```python
from build123d import *

# Parameters (mm, degrees)
SKETCH1_W           = 113
SKETCH1_H           = 98
BOSS_EXTRUDE1_DEPTH = 100
CUT_EXTRUDE1_DEPTH  = 130
CUT_EXTRUDE3_DEPTH  = 95
SKETCH4_W           = 113
SKETCH4_H           = 88.876192891
CUT_EXTRUDE4_DEPTH  = 95
BOSS_EXTRUDE4_DEPTH = 5
SKETCH7_W           = 36.687301185
SKETCH7_H           = 28.468155535
BOSS_EXTRUDE6_DEPTH = 25
SKETCH8_R           = 15
CUT_EXTRUDE5_DEPTH  = 25
FILLET1_R           = 20


with BuildPart() as part:
    # Sketch1 → Boss-Extrude1 (new body)
    with BuildSketch(Plane(origin=(0, 0, 0), x_dir=(1, 0, 0), z_dir=(0, 1, 0))):
        with Locations((9.126923077, -28.796153846)):
            Rectangle(SKETCH1_W, SKETCH1_H)
    extrude(amount=-BOSS_EXTRUDE1_DEPTH)

    # Sketch2 → Cut-Extrude1 (cut)
    with BuildSketch(Plane(origin=(65.626923077, 0, 0), x_dir=(0, 0, -1), z_dir=(1, 0, 0))):
        Polygon((20.203846154, 0), (-77.796153846, -50), (-77.796153846, 0), align=None)
    extrude(amount=-CUT_EXTRUDE1_DEPTH, mode=Mode.SUBTRACT)

    # Sketch3 → Cut-Extrude3 (cut)
    with BuildSketch(Plane(origin=(0, 0, -20.203846154), x_dir=(-1, 0, 0), z_dir=(0, 0, -1))):
        Polygon((-34.397311681, 0), (47.373076923, -88.732184402), (47.373076923, 0), align=None)
    extrude(amount=-CUT_EXTRUDE3_DEPTH, mode=Mode.SUBTRACT)

    # Sketch4 → Cut-Extrude4 (cut)
    with BuildSketch(Plane(origin=(0, 0, 0), x_dir=(1, 0, 0), z_dir=(0, 1, 0))):
        with Locations((9.126923077, -30.184844361)):
            Rectangle(SKETCH4_W, SKETCH4_H)
    extrude(amount=-CUT_EXTRUDE4_DEPTH, mode=Mode.SUBTRACT)

    # Sketch6 → Boss-Extrude4 (add)
    with BuildSketch(Plane(origin=(65.626923077, 0, 0), x_dir=(0, 0, -1), z_dir=(1, 0, 0))):
        Polygon((14.253252085, -95), (14.253252085, -3.036017382), (-74.622940806, -58.738358676), (-74.622940806, -95), align=None)
    extrude(amount=-BOSS_EXTRUDE4_DEPTH)

    # Sketch7 → Boss-Extrude6 (add)
    with BuildSketch(Plane(origin=(0, -95, 0), x_dir=(1, 0, 0), z_dir=(0, 1, 0))):
        with Locations((42.283272485, 0.019174318)):
            Rectangle(SKETCH7_W, SKETCH7_H)
    extrude(amount=BOSS_EXTRUDE6_DEPTH)

    # Sketch8 → Cut-Extrude5 (cut)
    with BuildSketch(Plane.XY.offset(77.796153846)):
        with Locations((-26.771199052, -75)):
            Circle(SKETCH8_R)
    extrude(amount=-CUT_EXTRUDE5_DEPTH, mode=Mode.SUBTRACT)

    # Fillet1
    # the kernel refuses this fillet: 20 mm, written as the material it takes off along each edge
    with BuildSketch(Plane(origin=(-47.373076923, -25.745870671, 30.258060361), x_dir=(0, -0.8907618697082329, -0.454470341687874), z_dir=(0, -0.45447034168787404, 0.890761869708233))) as fillet1_piece_1:
        with BuildLine():
            CenterArc((FILLET1_R, FILLET1_R), FILLET1_R, 180, 90)
            Line((0, FILLET1_R), (0, 0))
            Line((0, 0), (FILLET1_R, 0))
        make_face()
    extrude(amount=103.367903479, mode=Mode.SUBTRACT)


solid = part.part
```
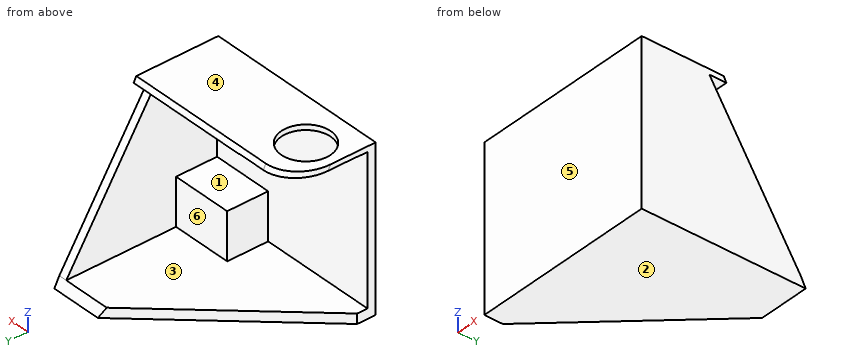
Geometry: final body of the model. Coordinates: model frame, mm. Face numbers are marked on the shaded views. A direction names the side the tool comes from. Round coordinates to 2 decimals unless told otherwise and drop trailing zeros. Order: outer loops, then holes, each group sorted by start corner. A loop starts at its lowest first (then second) coordinate and runs counter-clockwise, first axis right, second up. Notation, with made-up numbers: (37.25, 67.25) -> (70.25, 67.25) arc R18 ccw to (70.25, 84.25) -> close; hole circle Ø8 at (-12, 16). An arc over 180 degrees is marked (long way). Use one line per item in the form item = value. Start each with the question number.
1. Cut plane B-B (x = -31). Return the cut outline in (y, z).
2. Cut plane A-A (y = -75). Return the cut outline in (x, z), then the cut area to 3 significant figures.
3. Reachability of the marked faces 1 and 2 from +Z, -Z, +X, -X, +Y, -Y: full face, straight path, thin tool, end or side. Return the list, or none.
4. Pin query (flat end, axial travel): pin 1 Ø2 at (x, z) = (-18, 17.5) entering from +Y; pin 2 Ø12 at (x, y) = (31, -33.5) entering from +Z; pin 3 Ø12 at (y, z) = (-21, 15) entering from -X. Return the tip coordinate at first contact, or that it passes through.
5. Draft query along Z for the marked faces 3, 4, 5 and 6. Return one class per face: pulls with the +Z half, pulls with the -Z half, needs draft (parallel to the pull), parting line crosses it, or undercut.
6. Cut plane C-C (x = 43.5). Return the cut outline in (y, z), then the cut area to 3 significant figures.
7. Line query: probe 1 along Z at (x, y) = (-42, -92); probe 2 along Z at (x, y) = (34, -78); probe 3 along Z at (x, y) = (28, -26). Output: solid intervals per line, ascending.
8. Cut plane D-D (z = 1). Return the cut outline in (x, y).
Solution:
q1.outline = (-100, -20.2) -> (-70.97, -20.2) -> (-70.97, -14.25) -> (-95, -14.25) -> (-95, 74.62) -> (-89.39, 74.62) -> (-89.39, 77.8) -> (-100, 77.8) -> close; (-60.61, 74.8) -> (-48.84, 74.8) -> (-50.37, 77.8) -> (-60.61, 77.8) -> close
q2.outline = (-47.37, 74.8) -> (-41.77, 74.8) -> (-41.77, 77.8) -> (-47.37, 77.8) -> close; (-34.72, -20.2) -> (65.63, -20.2) -> (65.63, 77.8) -> (-11.77, 77.8) -> (-11.77, 74.62) -> (60.63, 74.62) -> (60.63, 14.21) -> (23.94, 14.21) -> (23.94, -14.25) -> (-34.72, -14.25) -> close
q2.area = 2,350 mm^2
q3.face_1 = -X, +Y
q3.face_2 = -Z, +X, -X, +Y, -Y
q4.pin_1 = -95
q4.pin_2 = -14.25
q4.pin_3 = 60.63
q5.face_3 = undercut
q5.face_4 = pulls with the +Z half
q5.face_5 = needs draft
q5.face_6 = undercut
q6.outline = (-100, -20.2) -> (0, -20.2) -> (-3.04, -14.25) -> (-70, -14.25) -> (-70, 14.21) -> (-95, 14.21) -> (-95, 74.62) -> (-48.38, 74.62) -> (-50, 77.8) -> (-100, 77.8) -> close
q6.area = 1,900 mm^2
q7.probe_1 = -20.2 to -14.25, 74.62 to 77.8
q7.probe_2 = -20.2 to 14.21, 74.62 to 77.8
q7.probe_3 = -20.2 to -14.25
q8.outline = (-47.37, -100) -> (65.63, -100) -> (65.63, -12.6) -> (60.63, -12.6) -> (60.63, -70) -> (23.94, -70) -> (23.94, -95) -> (-47.37, -95) -> close
